Verification items for the finished model (mm, model axes). Face numbers are marked on the shaded views. Round coordinates to 2 decimals unless told otherwise and drop trailing zeros. Write each loop counter-clockwise with the first axis right and the second up, starting at its lowest first coordinate (ties: lowest second). Pieces come first, ordered by that corner, then holes. Notation, with made-up numbers: (-39.75, 55) - (-0.75, 55) arc R30 cw to (-0.75, 79) - close; hole circle Ø2 at (52, -7.75). An arc over 180 degrees is marked (long way). Answer as a JSON object with one key per item and string values.
```python
from build123d import *

# Parameters (mm, degrees)
SKETCH_1_W          = 14
SKETCH_1_H          = 7
EXTRUDE_1_DEPTH     = 7
SKETCH_2_R          = 1.7
CUT_EXTRUDE_1_DEPTH = 6
CUT_EXTRUDE_1_DRAFT = -2


with BuildPart() as part:
    # Эскиз1 → Бобышка-Вытянуть1 (new body)
    with BuildSketch(Plane(origin=(0, 66.754264805, 0), x_dir=(-1, 0, 0), z_dir=(0, 0, 1))):
        with Locations((0, 66.754264805)):
            Rectangle(SKETCH_1_W, SKETCH_1_H)
    extrude(amount=EXTRUDE_1_DEPTH)


with BuildPart() as cut_extrude_1_tool:
    # Эскиз2 → Вырез-Вытянуть1 (with draft: the straight prism first)
    with BuildSketch(Plane.XY.offset(7)):
        Circle(SKETCH_2_R)
    extrude(amount=-CUT_EXTRUDE_1_DEPTH)
    # Вырез-Вытянуть1: the draft: its side faces are tilted about the plane it starts from
    cut_extrude_1_sides = [cut_extrude_1_tool.faces().sort_by_distance(p)[0] for p in [
        (-1.7, 0, 4),
    ]]
    draft(cut_extrude_1_sides, Plane.XY.offset(7), CUT_EXTRUDE_1_DRAFT)


with BuildPart() as part_1:
    add(part.part)

    # Вырез-Вытянуть1: cut by cut_extrude_1_tool
    add(cut_extrude_1_tool.part, mode=Mode.SUBTRACT)


solid = part_1.part
```
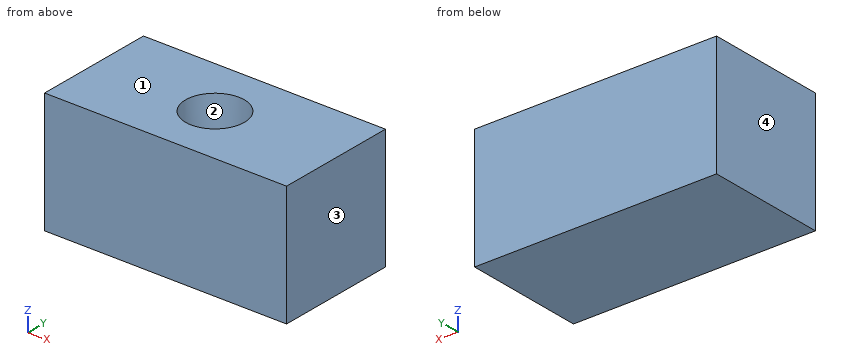
Q1. Section check D-D, the plane z = 2.25. Record the cut outline in (x, y), then the cut area to 3 significant figures.
Geometry check:
{"outline": "(-7, -3.5) - (7, -3.5) - (7, 3.5) - (-7, 3.5) - close; hole circle Ø3.07 at (0, 0)", "area": "90.6 mm2"}
Q2. Section check B-B, the plane y = 0. Record the cut outline in (x, z).
Geometry check:
{"outline": "(-7, 0) - (7, 0) - (7, 7) - (1.7, 7) - (1.49, 1) - (-1.49, 1) - (-1.7, 7) - (-7, 7) - close"}
Q3. Section check C-C, the plane z = 5.5. Record the cut outline in (x, y).
Geometry check:
{"outline": "(-7, -3.5) - (7, -3.5) - (7, 3.5) - (-7, 3.5) - close; hole circle Ø3.3 at (0, 0)"}
Q4. Section check A-A, the plane x = 0. Record the cut outline in (y, z), then the cut area to 3 significant figures.
Geometry check:
{"outline": "(-3.5, 0) - (3.5, 0) - (3.5, 7) - (1.7, 7) - (1.49, 1) - (-1.49, 1) - (-1.7, 7) - (-3.5, 7) - close", "area": "29.9 mm2"}
Q5. Material ranges on line 1 along X through (y, z) = (1, 2.5); line 2 along Y through (x, z) = (0.5, 2); line 3 along X through (y, z) = (-0.75, 2.5), recorded low to high. Write a range as [from, to].
Geometry check:
{"line 1": "x = [-7, -1.17], [1.17, 7]", "line 2": "y = [-3.5, -1.44], [1.44, 3.5]", "line 3": "x = [-7, -1.35], [1.35, 7]"}
Q6. Release check for a two-part mould opening along X. For the marked faces 1, 2, 3 and 4 record: released by +X, released by -X, zero draft, split by the parting line, or undercut.
Geometry check:
{"face 1": "zero draft", "face 2": "undercut", "face 3": "released by +X", "face 4": "released by -X"}
Q7. Gauge pin test, flat end, axial feed: P1, Ø0.9, axis at x = 0.5, y = -0.5, coming from the +Z side. Record the tip position at first contact, or that the pin passes through.
Geometry check:
{"P1": "stops at z = 1"}
